For this review, take the finished solid that the model builds, in its own axes (mm). A direction names the side the tool comes from. Coordinates: 2 decimals unless noted, no trailing zeros. Write each loop counter-clockwise with the first axis right and the second up, starting at its lowest first coordinate (ties: lowest second). Pieces come first, ordered by that corner, then holes. Notation, with made-up numbers: M -17,87 L 31,87 A24 cw 31,110 Z; hole C 37,77.25 d5. An arc over 180 degrees is marked long. One line per question, with ' | ' between items.
from build123d import *

# Parameters (mm, degrees)
F0_W      = 40
F0_H      = 40
F0_R      = 1.6
F1_DEPTH  = 1
F2_W      = 9.7
F2_H      = 9.6
F3_DEPTH  = 11.4
F4_R      = 3.4
F5_DEPTH  = 19.9
F6_R      = 8.1
F7_DEPTH  = 16
F8_W      = 14
F8_H      = 6
F9_DEPTH  = 5
F10_W     = 8.2
F10_H     = 20.2
F11_DEPTH = 10.5
F12_W     = 14
F12_H     = 10.1
F13_DEPTH = 11.5


with BuildPart() as f1:
    # F0 (on Top) → F1 (new body)
    with BuildSketch(Plane.XY):
        Rectangle(F0_W, F0_H)
        with Locations((-8.8, -17.4)):
            Circle(F0_R, mode=Mode.SUBTRACT)
        with Locations((15.2, -17.4)):
            Circle(F0_R, mode=Mode.SUBTRACT)
        with Locations((-6, 17.4)):
            Circle(F0_R, mode=Mode.SUBTRACT)
        with Locations((15.2, 17.4)):
            Circle(F0_R, mode=Mode.SUBTRACT)
    extrude(amount=F1_DEPTH)

    # F2 (on face) → F3 (join)
    with BuildSketch(Plane.XY.offset(1)):
        with Locations((15.15, -8.9)):
            Rectangle(F2_W, F2_H)
    extrude(amount=F3_DEPTH)

    # F4 (on face) → F5 (join)
    with BuildSketch(Plane.YZ.offset(20)):
        with Locations((-8.9, 7.6)):
            Circle(F4_R)
    extrude(amount=F5_DEPTH)

    # F6 (on face) → F7 (join)
    with BuildSketch(Plane.XY.offset(1)):
        with Locations((5.1, 10.4)):
            Circle(F6_R)
    extrude(amount=F7_DEPTH)

    # F8 (on face) → F9 (join)
    with BuildSketch(Plane.XY.offset(1)):
        with Locations((-15.6, 15.5)):
            Rectangle(F8_W, F8_H)
    extrude(amount=F9_DEPTH)

    # F10 (on face) → F11 (join)
    with BuildSketch(Plane.XY.offset(1)):
        with Locations((-15.9, -7.7)):
            Rectangle(F10_W, F10_H)
    extrude(amount=F11_DEPTH)

    # F12 (on face) → F13 (join)
    with BuildSketch(Plane.XY.offset(1)):
        with Locations((-13, 7.45)):
            Rectangle(F12_W, F12_H)
    extrude(amount=F13_DEPTH)


solid = f1.part
1. Take a section at D-D on y = -8.9. State the section outline as (x, z) points.
Computed values:
outline: M -20,0 L 20,0 L 20,4.2 L 39.9,4.2 L 39.9,11 L 20,11 L 20,12.4 L 10.3,12.4 L 10.3,1 L -11.8,1 L -11.8,11.5 L -20,11.5 Z
2. Clearance check with flat-ended pins moving along their axes: P1, Ø1.5, axis at y = -7, z = 7.5, coming from the -X side; P2, Ø6, axis at x = -12.5, z = 9.5, coming from the +Y side; P3, Ø5, axis at y = 7.5, z = 7, coming from the +X side. State where each tip first meets the part, or that it passes through.
Computed values:
P1: stops at x = -20 | P2: stops at y = 12.5 | P3: stops at x = 13.19
3. Draft analysis for pull direction X (two halves, no side actions). For faces 5 (the flat face through (-8.6, 15, 3)), 6 (the flat face through (10.3, -9, 7)), 7 (the flat face through (-16, 18.5, 3)), 8 (the flat face through (-22.6, 15, 3)), state which applies: pulls with the +X half, pulls with the -X half, needs draft (parallel to the pull), parting line crosses it, or undercut.
Computed values:
face 5: undercut | face 6: undercut | face 7: needs draft | face 8: pulls with the -X half
4. For line 1 along Y through (x, z) = (15.2, 0.5); line 2 along Y through (x, z) = (-8.8, 0.45); line 3 along Y through (x, z) = (-12, 7.75), list the stretches that pass through material, from the lowest coordinate up.
Computed values:
line 1: y = -20 to -19, -15.8 to 15.8, 19 to 20 | line 2: y = -20 to -19, -15.8 to 20 | line 3: y = -17.8 to 12.5
5. Take a section at C-C on y = 17.4. State the section outline as (x, z) points, plus the area to 3 significant figures.
Computed values:
outline: M -22.6,1 L -20,1 L -20,0 L -7.6,0 L -7.6,1 L -8.6,1 L -8.6,6 L -22.6,6 Z; M -4.4,0 L 13.6,0 L 13.6,1 L 9.18,1 L 9.18,17 L 1.02,17 L 1.02,1 L -4.4,1 Z; M 16.8,0 L 20,0 L 20,1 L 16.8,1 Z | area: 234 mm2
6. Machinability: for faces 1 (the flat face through (15, -4.1, 7)), 2 (the flat face through (-16, 16, 6)), 3 (the flat face through (-16, -8, 11.5)), 4 (the flat face through (15, -9, 12.4)), which of the approach directions +Z, -Z, +X, -X, +Y, -Y give a long, thin tool a straight path to every point of the face, cutting with its end or side? Answer none if there is none.
Computed values:
face 1: +Z, +X | face 2: +Z, -X, +Y | face 3: +Z, -X, -Y | face 4: +Z, +X, -X, -Y
7. Take a section at B-B on x = 15.2. State the section outline as (y, z) points.
Computed values:
outline: M -20,0 L -19,0 L -19,1 L -20,1 Z; M -15.8,0 L 15.8,0 L 15.8,1 L -4.1,1 L -4.1,12.4 L -13.7,12.4 L -13.7,1 L -15.8,1 Z; M 19,0 L 20,0 L 20,1 L 19,1 Z
8. Take a section at A-A on z = 7.6. State the section outline as (x, y) points, plus the area to 3 significant figures.
Computed values:
outline: M -20,-17.8 L -11.8,-17.8 L -11.8,2.4 L -6,2.4 L -6,12.5 L -20,12.5 Z; C 5.1,10.4 d16.2; M 10.3,-13.7 L 20,-13.7 L 20,-12.3 L 39.9,-12.3 L 39.9,-5.5 L 20,-5.5 L 20,-4.1 L 10.3,-4.1 Z | area: 742 mm2
